Design review of the part shown in the three views and the two pictorial views. Dimensions are in mm from the part's minimum x, y and z. A direction names the side the tool comes from. Coordinates: 2 decimals unless noted, no trailing zeros. Loops run counter-clockwise (first coordinate to the right, second up) from the corner with the lowest first, then second, coordinate; pieces in that order, holes last. Notation, with made-up numbers: (-33.75, -19) - (-17.75, -19) arc R26 cw to (-17.75, 18) - close; hole circle Ø1 at (-25.5, 87.5). An arc over 180 degrees is marked (long way). One line per question, with ' | ' between items.
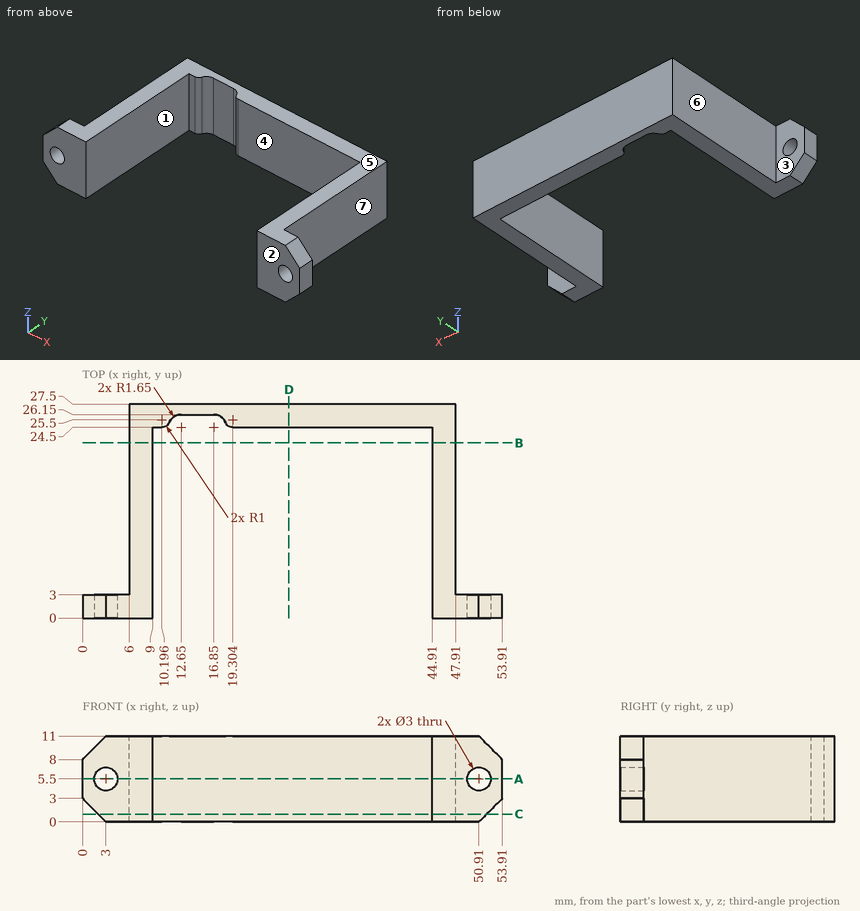
Q1. Tool access review of the marked faces 1, 2 and 3: name each direction out of +Z, -Z, +X, -X, +Y, -Y from which nothing blocks a thin tool from reaching the whole face with its end or side.
Returned:
face 1: +Z, -Z, -Y | face 2: +Z, -Z, +X, -X, -Y | face 3: +Z, -Z, -X, +Y
Q2. For pin 1 (3.5 mm diameter, centred on y = 19.5, z = 4, fed in from -X); pin 2 (1.8 mm diameter, centred on x = 2, z = 6, fed in from +Y); pin 3 (5 mm diameter, centred on x = 13.5, y = 15.5, fed in from -Z); pin 4 (4.5 mm diameter, centred on x = 14, z = 6.5, fed in from -Y), all flat-tipped, find the tip position at first contact; note any pin that passes through.
Returned:
pin 1: stops at x = 6 | pin 2: stops at y = 3 | pin 3: passes through | pin 4: stops at y = 25.88
Q3. Draft analysis for pull direction X (two halves, no side actions). For the marked faces 4, 5, 6 and 7, state which applies: +X half, -X half, draft (parallel to the pull), parting line (faces both ways), or undercut.
Returned:
face 4: undercut | face 5: draft | face 6: -X half | face 7: +X half
Q4. Take a section at C-C (z = 1). Give the boundary of the cut face in (x, y).
Returned:
outline: (2, 0) - (9, 0) - (9, 24.5) - (10.2, 24.5) arc R1 ccw to (11.12, 25.12) arc R1.65 cw to (12.65, 26.15) - (16.85, 26.15) arc R1.65 cw to (18.38, 25.12) arc R1 ccw to (19.3, 24.5) - (44.91, 24.5) - (44.91, 0) - (51.91, 0) - (51.91, 3) - (47.91, 3) - (47.91, 27.5) - (6, 27.5) - (6, 3) - (2, 3) - close
Q5. Take a section at D-D (x = 26.5). Give the boundary of the cut face in (y, z).
Returned:
outline: (24.5, 0) - (27.5, 0) - (27.5, 11) - (24.5, 11) - close
Q6. To check wall thickness, follow line 1 along Z through (x, y) = (50.91, 1.6); line 2 along X through (y, z) = (21.5, 4.5); line 3 along Y through (x, z) = (24, 1.25). State the ranges of each line that lie inside material, in increasing order.
Returned:
line 1: z = 0 to 4, 7 to 11 | line 2: x = 6 to 9, 44.91 to 47.91 | line 3: y = 24.5 to 27.5
Q7. Take a section at B-B (y = 22.5). Give the boundary of the cut face in (x, z), plus the area to 3 significant figures.
Returned:
outline: (6, 0) - (9, 0) - (9, 11) - (6, 11) - close; (44.91, 0) - (47.91, 0) - (47.91, 11) - (44.91, 11) - close | area: 66.0 mm²
Q8. Take a section at A-A (z = 5.5). Give the boundary of the cut face in (x, y), plus the area to 3 significant figures.
Returned:
outline: (0, 0) - (1.5, 0) - (1.5, 3) - (0, 3) - close; (4.5, 0) - (9, 0) - (9, 24.5) - (10.2, 24.5) arc R1 ccw to (11.12, 25.12) arc R1.65 cw to (12.65, 26.15) - (16.85, 26.15) arc R1.65 cw to (18.38, 25.12) arc R1 ccw to (19.3, 24.5) - (44.91, 24.5) - (44.91, 0) - (49.41, 0) - (49.41, 3) - (47.91, 3) - (47.91, 27.5) - (6, 27.5) - (6, 3) - (4.5, 3) - close; (52.41, 0) - (53.91, 0) - (53.91, 3) - (52.41, 3) - close | area: 279 mm²
